Geometry: final body of the model. Coordinates: model frame, mm. A direction names the side the tool comes from. Round coordinates to 2 decimals unless told otherwise and drop trailing zeros. Write each loop counter-clockwise with the first axis right and the second up, starting at its lowest first coordinate (ties: lowest second). Pieces come first, ordered by that corner, then holes. Notation, with made-up numbers: (-6, 89) -> (34, 89) arc R28 ccw to (34, 118) -> close; hole circle Ø5 at (19, -6). An arc over 180 degrees is marked (long way). Use one line per item in the form item = value. Start each with the question number.
1. Pin query (flat end, axial travel): pin 1 Ø9.5 at (x, z) = (0, 108.5) entering from +Y; pin 2 Ø1 at (x, z) = (-4.5, -2.5) entering from -Y; pin 3 Ø3 at (x, z) = (1, -25) entering from -Y; pin 4 Ø3 at (x, y) = (-7, 9.5) entering from +Z. Return the tip coordinate at first contact, or that it passes through.
2. Line query: L1, parallel to Z at x = 4.5, y = 2; L2, parallel to Z at x = -7, y = 23; L3, parallel to X at y = 38, z = -84. Output: solid intervals per line, ascending.
3. Cut plane A-A, the plane z = -104. Return the cut outline in (x, y), plus the area to 3 significant figures.
4. Cut plane D-D, the plane y = 38. Return the cut outline in (x, z), plus the area to 3 significant figures.
5. Cut plane B-B, the plane y = 23. Return the cut outline in (x, z), plus the area to 3 significant figures.
6. Cut plane C-C, the plane x = -4.25. Return the cut outline in (y, z), plus the area to 3 significant figures.
7. Draft query along Y for faces 1 (the face through (4.3, 3, -111.6)), 2 (the face through (0, 0, 111)), 3 (the face through (-2, 38, 119)), 4 (the face through (0, 3, 107)). Return one class per face: pulls with the +Y half, pulls with the -Y half, needs draft (parallel to the pull), parting line crosses it, or undercut.
8. Reachability of faces 5 (the face through (-2, 18, 107)), 6 (the face through (-2, 38, -119)), 7 (the face through (0, 0, -112)) from +Z, -Z, +X, -X, +Y, -Y: full face, straight path, thin tool, end or side. Return the list, or none.
```python
from build123d import *

# Parameters (mm, degrees)
SK_P01_FOOT_W  = 20
SK_P01_FOOT_H  = 19
P01_FOOT_DEPTH = 3
SK_P02_FOOT_W  = 20
SK_P02_FOOT_H  = 19
P02_FOOT_DEPTH = 3
P03_LEG_START  = 3
SK_P03_LEG_R   = 6
P03_LEG_DEPTH  = 35
P04_LEG_START  = 3
SK_P04_LEG_R   = 6
P04_LEG_DEPTH  = 35
P05_GRIP_START = -119
SK_P05_GRIP_R  = 8
P05_GRIP_DEPTH = 238


with BuildPart() as part:
    # SK_P01_Foot → P01_Foot (new body)
    with BuildSketch(Plane(origin=(0, 0, 0), x_dir=(1, 0, 0), z_dir=(0, 1, 0))):
        with Locations((0, -111.5)):
            Rectangle(SK_P01_FOOT_W, SK_P01_FOOT_H)
    extrude(amount=P01_FOOT_DEPTH)

    # SK_P03_Leg → P03_Leg (add)
    with BuildSketch(Plane(origin=(0, 0, 0), x_dir=(1, 0, 0), z_dir=(0, 1, 0)).offset(P03_LEG_START)):
        with Locations(Location((-2, -113, 0), (0, 0, 270))):
            Circle(SK_P03_LEG_R)
    extrude(amount=P03_LEG_DEPTH)



with BuildPart() as body_2:
    # SK_P02_Foot → P02_Foot (new body)
    with BuildSketch(Plane(origin=(0, 0, 0), x_dir=(1, 0, 0), z_dir=(0, 1, 0))):
        with Locations((0, 111.5)):
            Rectangle(SK_P02_FOOT_W, SK_P02_FOOT_H)
    extrude(amount=P02_FOOT_DEPTH)

    # SK_P04_Leg → P04_Leg (add)
    with BuildSketch(Plane(origin=(0, 0, 0), x_dir=(1, 0, 0), z_dir=(0, 1, 0)).offset(P04_LEG_START)):
        with Locations(Location((-2, 113, 0), (0, 0, 270))):
            Circle(SK_P04_LEG_R)
    extrude(amount=P04_LEG_DEPTH)


with BuildPart() as part_1:
    add(part.part)

    add(body_2.part)  # P05_Grip merges body 2
    # SK_P05_Grip → P05_Grip (add)
    with BuildSketch(Plane.XY.offset(P05_GRIP_START)):
        with Locations(Location((-2, 38, 0), (0, 0, 270))):
            Circle(SK_P05_GRIP_R)
    extrude(amount=P05_GRIP_DEPTH)


solid = part_1.part
```
Outcome:
q1.pin_1 = 46
q1.pin_2 = 30.25
q1.pin_3 = 30.14
q1.pin_4 = 117.87
q2.L1 = -121 to -102, 102 to 121
q2.L2 = -116.32 to -109.68, 109.68 to 116.32
q2.L3 = -10 to 6
q3.outline = (-10, 0) -> (10, 0) -> (10, 3) -> (-10, 3) -> close; circle Ø16 at (-2, 38)
q3.area = 261 mm^2
q4.outline = (-10, -119) -> (6, -119) -> (6, 119) -> (-10, 119) -> close
q4.area = 3,810 mm^2
q5.outline = circle Ø12 at (-2, -113); circle Ø12 at (-2, 113)
q5.area = 226 mm^2
q6.outline = (0, -121) -> (3, -121) -> (3, -118.56) -> (30.32, -118.56) -> (30.32, -119) -> (45.68, -119) -> (45.68, 119) -> (30.32, 119) -> (30.32, 118.56) -> (3, 118.56) -> (3, 121) -> (0, 121) -> (0, 102) -> (3, 102) -> (3, 107.44) -> (30.32, 107.44) -> (30.32, -107.44) -> (3, -107.44) -> (3, -102) -> (0, -102) -> close
q6.area = 4,380 mm^2
q7.face_1 = undercut
q7.face_2 = pulls with the -Y half
q7.face_3 = needs draft
q7.face_4 = undercut
q8.face_5 = none
q8.face_6 = -Z, +X, -X, +Y
q8.face_7 = +Z, -Z, +X, -X, -Y
